Can you work these out from the model? Positions are in its coordinate system, mm. A direction names the side the tool comes from. Coordinates: 2 decimals unless noted, no trailing zeros. Loops run counter-clockwise (first coordinate to the right, second up) from the corner with the lowest first, then second, coordinate; pieces in that order, holes last. Notation, with made-up numbers: M 40.25,78.5 L 86.25,78.5 A16 cw 86.25,86.5 Z; hole C 8,-33 d7. An arc over 180 degrees is marked long. Return JSON: item names as keys, results as strings. Group by question number.
```python
from build123d import *

# Parameters (mm, degrees)
SKETCH1_R           = 30
BOSS_EXTRUDE1_DEPTH = 3.6
SKETCH2_R           = 25
BOSS_EXTRUDE2_DEPTH = 4.6
SKETCH3_R           = 20
BOSS_EXTRUDE3_DEPTH = 6
CUT_EXTRUDE1_REACH  = 46.74
SKETCH4_R           = 2.1
CHAMFER1_SIZE       = 2


with BuildPart() as part:
    # Sketch1 → Boss-Extrude1 (new body)
    with BuildSketch(Plane(origin=(0, 0, 0), x_dir=(1, 0, 0), z_dir=(0, 1, 0))):
        with Locations(Location((0, 0, 0), (0, 0, 270))):
            Circle(SKETCH1_R)
    extrude(amount=BOSS_EXTRUDE1_DEPTH)

    # Sketch2 → Boss-Extrude2 (add)
    with BuildSketch(Plane(origin=(0, 3.6, 0), x_dir=(1, 0, 0), z_dir=(0, 1, 0))):
        with Locations(Location((0, 0, 0), (0, 0, 270))):
            Circle(SKETCH2_R)
    extrude(amount=BOSS_EXTRUDE2_DEPTH)

    # Sketch3 → Boss-Extrude3 (add)
    with BuildSketch(Plane(origin=(0, 8.2, 0), x_dir=(1, 0, 0), z_dir=(0, 1, 0))):
        with Locations(Location((0, 0, 0), (0, 0, 270))):
            Circle(SKETCH3_R)
    extrude(amount=BOSS_EXTRUDE3_DEPTH)

    # Sketch4 → Cut-Extrude1 (cut, up to next)
    with BuildSketch(Plane(origin=(0, 14.2, 0), x_dir=(1, 0, 0), z_dir=(0, 1, 0)), mode=Mode.PRIVATE) as cut_extrude1_sk1:
        with Locations(Location((0, 15, 0), (0, 0, 270))):
            Circle(SKETCH4_R)
    cut_extrude1_tool1 = extrude(cut_extrude1_sk1.sketch, amount=-CUT_EXTRUDE1_REACH, mode=Mode.PRIVATE) & part.part
    # Sketch4 → Cut-Extrude1 (cut, up to next)
    with BuildSketch(Plane(origin=(0, 14.2, 0), x_dir=(1, 0, 0), z_dir=(0, 1, 0)), mode=Mode.PRIVATE) as cut_extrude1_sk2:
        with Locations(Location((12.990381057, -7.5, 0), (0, 0, 270))):
            Circle(SKETCH4_R)
    cut_extrude1_tool2 = extrude(cut_extrude1_sk2.sketch, amount=-CUT_EXTRUDE1_REACH, mode=Mode.PRIVATE) & part.part
    # Sketch4 → Cut-Extrude1 (cut, up to next)
    with BuildSketch(Plane(origin=(0, 14.2, 0), x_dir=(1, 0, 0), z_dir=(0, 1, 0)), mode=Mode.PRIVATE) as cut_extrude1_sk3:
        with Locations(Location((-12.990381057, -7.5, 0), (0, 0, 270))):
            Circle(SKETCH4_R)
    cut_extrude1_tool3 = extrude(cut_extrude1_sk3.sketch, amount=-CUT_EXTRUDE1_REACH, mode=Mode.PRIVATE) & part.part
    add(cut_extrude1_tool1.solids().sort_by_distance((0, 14.2, -15))[0], mode=Mode.SUBTRACT)
    add(cut_extrude1_tool2.solids().sort_by_distance((12.990381, 14.2, 7.5))[0], mode=Mode.SUBTRACT)
    add(cut_extrude1_tool3.solids().sort_by_distance((-12.990381, 14.2, 7.5))[0], mode=Mode.SUBTRACT)

    # Chamfer1
    chamfer1_edges = [part.edges().sort_by_distance(p)[0] for p in [
        (0, 0, -17.1),
        (12.990381057, 0, 5.4),
        (-12.990381057, 0, 5.4),
    ]]
    chamfer(chamfer1_edges, length=CHAMFER1_SIZE)


solid = part.part
```
1) Suppose I cut it at A-A, the plane x = 0. List the corners of the cut face in (y, z) for me.
2) Suppose I cut it at C-C, the plane z = 7.5. List the corners of the cut face in (x, y) for me.
3) Suppose I cut it at D-D, the plane z = 0. List the corners of the cut face in (x, y) for me, then the cut area to 3 significant figures.
4) For faces 1 (the face through (0, 14.2, 0)), 2 (the face through (25, 3.6, -7)), which set-ups out of +Z, -Z, +X, -X, +Y, -Y let a thin tool reach every point of the face, with its end or its side?
5) If we mould it in two halves opening along Z, with no side actions, what happens to faces 3 (the face through (-1.278, 8.185, -16.666)), 4 (the face through (17, 8.2, -11)), 5 (the face through (7.509, 5.868, 23.846))? For each: +Z half, -Z half, draft (parallel to the pull), parting line (faces both ways), or undercut.
6) For pin 1 (6 mm diameter, centred on y = 9.5, z = -5, fed in from +X); pin 2 (6.5 mm diameter, centred on x = 0, z = -15, fed in from -Y); pin 3 (2.5 mm diameter, centred on x = 12.99, z = 7.5, fed in from -Y); pin 4 (2 mm diameter, centred on y = 4, z = -10.5, fed in from +X), each with a flat end and sliding along its axis, tell me the tip position at first contact or that it passes through.
7) Suppose I cut it at B-B, the plane z = -15. List the corners of the cut face in (x, y) for me, then the cut area to 3 significant figures.
8) If I drill on line 1 (X direction, y = 5.25, z = -15); line 2 (Y direction, x = 18.5, z = 18.5); line 3 (X direction, y = 8.5, z = -15), over which ranges is the centre line in solid material (lowest first)? Write a range as from..to.
Returned:
{
 "1": {"outline": "M 0,-30 L 3.6,-30 L 3.6,-25 L 8.2,-25 L 8.2,-20 L 14.2,-20 L 14.2,-17.1 L 2,-17.1 L 0,-19.1 Z; M 0,-10.9 L 2,-12.9 L 14.2,-12.9 L 14.2,20 L 8.2,20 L 8.2,25 L 3.6,25 L 3.6,30 L 0,30 Z"},
 "2": {"outline": "M -29.05,0 L -17.09,0 L -15.09,2 L -15.09,14.2 L -18.54,14.2 L -18.54,8.2 L -23.85,8.2 L -23.85,3.6 L -29.05,3.6 Z; M -10.89,2 L -8.89,0 L 8.89,0 L 10.89,2 L 10.89,14.2 L -10.89,14.2 Z; M 15.09,2 L 17.09,0 L 29.05,0 L 29.05,3.6 L 23.85,3.6 L 23.85,8.2 L 18.54,8.2 L 18.54,14.2 L 15.09,14.2 Z"},
 "3": {"outline": "M -30,0 L 30,0 L 30,3.6 L 25,3.6 L 25,8.2 L 20,8.2 L 20,14.2 L -20,14.2 L -20,8.2 L -25,8.2 L -25,3.6 L -30,3.6 Z", "area": "686 mm²"},
 "4": {"face 1": "+Z, -Z, +X, -X, +Y", "face 2": "+Y"},
 "5": {"face 3": "undercut", "face 4": "draft", "face 5": "parting line"},
 "6": {"pin 1": "stops at x = 24.89", "pin 2": "stops at y = 0.85", "pin 3": "passes through", "pin 4": "stops at x = 28.43"},
 "7": {"outline": "M -25.98,0 L -4.1,0 L -2.1,2 L -2.1,14.2 L -13.23,14.2 L -13.23,8.2 L -20,8.2 L -20,3.6 L -25.98,3.6 Z; M 2.1,2 L 4.1,0 L 25.98,0 L 25.98,3.6 L 20,3.6 L 20,8.2 L 13.23,8.2 L 13.23,14.2 L 2.1,14.2 Z", "area": "466 mm²"},
 "8": {"line 1": "x = -20..-2.1, 2.1..20", "line 2": "y = 0..3.6", "line 3": "x = -13.23..-2.1, 2.1..13.23"}
}
